```python
from build123d import *

# Parameters (mm, degrees)
BASPROSKE_W        = 10
BASPROSKE_H        = 18
TOOTHCUT_DEPTH     = 28.349588662
TEETHCUTS_COUNT    = 10
TEETHCUTS_ANGLE    = 324
HUBNEAONESKE_R     = 10
HUBNEARONE_DEPTH   = 10.0000508
BORSKE_R           = 3.5
BORE_DEPTH         = 20.0000508
CUT_EXTRUDE1_DEPTH = 6
SKETCH2_R          = 4
CUT_EXTRUDE2_DEPTH = 29.581121206
SKETCH3_R          = 2.25
CUT_EXTRUDE3_DEPTH = 27.8492101


with BuildPart() as part:
    # BasProSke → Base-Revolve (revolve)
    with BuildSketch(Plane(origin=(0, 0, 0), x_dir=(1, 0, 0), z_dir=(0, 1, 0)), mode=Mode.PRIVATE) as base_revolve_sk:
        with Locations((5, 9)):
            Rectangle(BASPROSKE_W, BASPROSKE_H)
    revolve(base_revolve_sk.sketch.rotate(Axis((-10, 0, 0), (1, 0, 0)), 180), axis=Axis((-10, 0, 0), (1, 0, 0)))

    # TooCutSke → ToothCut (cut, through all)
    with BuildSketch(Plane(origin=(0, 0, 0), x_dir=(0, 0, -1), z_dir=(1, 0, 0))):
        with BuildLine():
            ThreePointArc((1.768949054, 11.109042274), (0, 11.249), (-1.768949054, 11.109042274))
            ThreePointArc((-1.768949054, 11.109042274), (-2.508977513, 14.741789417), (-5.242576524, 17.246171649))
            ThreePointArc((-5.242576524, 17.246171649), (0, 18.0254), (5.242576524, 17.246171649))
            ThreePointArc((5.242576524, 17.246171649), (2.508977513, 14.741789417), (1.768949054, 11.109042274))
        make_face()
    toothcut = extrude(amount=TOOTHCUT_DEPTH, mode=Mode.SUBTRACT)

    # TeethCuts: ToothCut ×10 about axis
    teethcuts_axis = Axis((-10, 0, 0), (1, 0, 0))
    for i in range(1, TEETHCUTS_COUNT):
        add(toothcut.rotate(teethcuts_axis, i * TEETHCUTS_ANGLE / (TEETHCUTS_COUNT - 1)), mode=Mode.SUBTRACT)

    # HubNeaOneSke → HubNearOne (add)
    with BuildSketch(Plane.ZY):
        with Locations(Location((0, 0, 0), (0, 0, 180))):
            Circle(HUBNEAONESKE_R)
    extrude(amount=HUBNEARONE_DEPTH)

    # BorSke → Bore (cut, symmetric)
    with BuildSketch(Plane(origin=(0, 0, 0), x_dir=(0, 0, -1), z_dir=(1, 0, 0))):
        with Locations(Location((0, 0, 0), (0, 0, 180))):
            Circle(BORSKE_R)
    extrude(amount=BORE_DEPTH, both=True, mode=Mode.SUBTRACT)

    # Sketch1 → Cut-Extrude1 (cut)
    with BuildSketch(Plane.ZY.offset(10.0000508)):
        Polygon((7.794228634, 0), (3.897114317, 6.75), (-3.897114317, 6.75), (-7.794228634, 0), (-3.897114317, -6.75), (3.897114317, -6.75), align=None)
    extrude(amount=-CUT_EXTRUDE1_DEPTH, mode=Mode.SUBTRACT)

    # Sketch2 → Cut-Extrude2 (cut, through all)
    with BuildSketch(Plane.ZY.offset(4.0000508)):
        Circle(SKETCH2_R)
    extrude(amount=-CUT_EXTRUDE2_DEPTH, mode=Mode.SUBTRACT)

    # Sketch3 → Cut-Extrude3 (cut, through all)
    with BuildSketch(Plane(origin=(0, 0, 0), x_dir=(1, 0, 0), z_dir=(0, 1, 0))):
        with Locations(Location((-7.0000508, 0, 0), (0, 0, 270))):
            Circle(SKETCH3_R)
    extrude(amount=-CUT_EXTRUDE3_DEPTH, mode=Mode.SUBTRACT)


solid = part.part
```
Could you check a few things on this model? Use its own coordinates, in mm. Round coordinates to 2 decimals unless told otherwise and drop trailing zeros. Loops run counter-clockwise (first coordinate to the right, second up) from the corner with the lowest first, then second, coordinate; pieces in that order, holes last. Notation, with made-up numbers: (61, 77) - (79, 77) arc R17 ccw to (79, 108) - close; hole circle Ø8 at (46, 58). An arc over 180 degrees is marked (long way). Answer in a Markdown table with one row per item. Add a question column.
(1) If we section it at A-A (z = 0.5): Please give me the cut outline in (x, y).
(2) If we section it at B-B (z = -13): Please give me the cut outline in (x, y), plus the area to 3 significant figures.
(3) I'm going to push flat-ended pins straight in: pin 1 (7 mm diameter, centred on y = 0, z = 0, fed in from +X); pin 2 (1 mm diameter, centred on x = -5.5, y = -7.5, fed in from +Z); pin 3 (6 mm diameter, centred on x = 2, z = -13, fed in from -Y); pin 4 (7 mm diameter, centred on x = -7, z = 0, fed in from -Y). Where does each tip first touch, or does it pass through?
(4) If we mould it in two halves opening along Y, with no side actions, what happens to faces 1 (the face through (4.93, 3.452, -10.706)), 2 (the face through (10, -0.2, 4.3)), 3 (the face through (-4.93, 9.76, 2.17))? For each: pulls with the +Y half, pulls with the -Y half, needs draft (parallel to the pull), parting line crosses it, or undercut.
(5) I need wall thicknesses on line 1 along X through (y, z) = (-8.1, 0); line 2 along Y through (x, z) = (4, -12.5); line 3 along Y through (x, z) = (1.5, -14). Which ranges of each line are inside material? Lowest first, please.
Model answer:
| question | item | result |
|---|---|---|
| 1 | outline | (-10, -9.99) - (-9.19, -9.99) - (-9.19, -6.75) - (-10, -6.75) - close; (-10, 6.75) - (-4, 6.75) - (-4, 3.97) - (10, 3.97) - (10, 11.24) - (0, 11.24) - (0, 9.99) - (-10, 9.99) - close; (-4.81, -9.99) - (0, -9.99) - (0, -11.24) - (10, -11.24) - (10, -3.97) - (-4, -3.97) - (-4, -6.75) - (-4.81, -6.75) - close |
| 2 | outline | (0, -10.99) - (10, -10.99) - (10, -6.69) - (0, -6.69) - close; (0, -2.26) - (10, -2.26) - (10, 2.26) - (0, 2.26) - close; (0, 6.69) - (10, 6.69) - (10, 10.99) - (0, 10.99) - close |
| 2 | area | 131 mm² |
| 3 | pin 1 | passes through |
| 3 | pin 2 | stops at z = 7.14 |
| 3 | pin 3 | stops at y = -10.99 |
| 3 | pin 4 | stops at y = -10 |
| 4 | face 1 | undercut |
| 4 | face 2 | needs draft |
| 4 | face 3 | parting line crosses it |
| 5 | line 1 | x = -10 to -9.25, -4.75 to 10 |
| 5 | line 2 | y = -10.95 to -6.26, -2.19 to 2.19, 6.26 to 10.95 |
| 5 | line 3 | y = -10.94 to -7.97, -2.28 to 2.28, 7.97 to 10.94 |
